Model file for the job. Use its own axes, mm. A direction names the side the tool comes from. Give positions to 0.01 mm unless a question says otherwise; leave off trailing zeros. Order: outer loops, then holes, each group sorted by start corner. A loop starts at its lowest first (then second) coordinate and runs counter-clockwise, first axis right, second up. Notation, with made-up numbers: M 87.25,36 L 114.25,36 A22 cw 114.25,59 Z; hole C 53.25,86 d3. An arc over 180 degrees is marked long. Return JSON: item names as keys, results as strings. Group by question number.
1. Wall check: probe 1 along Z at (x, y) = (55.5, 64); probe 2 along Y at (x, z) = (148.5, 54.5); probe 3 along Y at (x, z) = (10, 7.5). Give the ranges that are in metal, low to high. Write a range as [from, to].
2. Slice it at B-B on x = 24. List the corners of the cut face in (y, z), then the cut area to 3 significant figures.
3. Slice it at A-A on z = 68. List the corners of the cut face in (x, y), then the cut area to 3 significant figures.
4. Two-plate mould, pull along Y, no slides. Class faces 3 (the face through (92, 2, 8)), 4 (the face through (92, 0, 50)), 5 (the face through (92, 75, 98)): released by +Y, released by -Y, zero draft, split by the parting line, or undercut.
5. 3-axis set-ups, long thin cutter, end or side, ignore diameter. For faces 1 (the face through (92, 69, 96)), 2 (the face through (0, 73.2, 96.4)): which of +Z, -Z, +X, -X, +Y, -Y reach the whole face in a straight line?
6. Slice it at D-D on z = 89.5. List the corners of the cut face in (x, y).
7. Slice it at C-C on y = 94. List the corners of the cut face in (x, z).
Autodesk Inventor part; units mm, degrees
ref_plane "YZ Plane" through (0, 0, 0) normal (1, 0, 0) x (0, 1, 0)
ref_plane "XZ Plane" through (0, 0, 0) normal (0, 1, 0) x (-1, 0, 0)
ref_plane "XY Plane" through (0, 0, 0) normal (0, 0, 1) x (1, 0, 0)
sketch "Sketch1" plane through (0, 0, 0) normal (1, 0, 0) x (0, 1, 0)
  line L0 (0, 0) -> (147, 0)
  line L1 (147, 0) -> (147, 98)
  line L2 (147, 98) -> (0, 98)
  line L3 (0, 98) -> (0, 0)
  line L4 (2, 2) -> (145, 2)
  line L5 (145, 2) -> (145, 96)
  line L6 (145, 96) -> (2, 96)
  line L7 (2, 96) -> (2, 2)
  line L8 (137, 96) -> (135, 96)
  line L9 (135, 96) -> (135, 93)
  line L10 (135, 93) -> (137, 93)
  line L11 (137, 93) -> (137, 96)
  circle A0 centre (136, 90.1716) radius 3
  line L12 (135, 2) -> (133, 2)
  line L13 (133, 2) -> (133, 5)
  line L14 (133, 5) -> (135, 5)
  line L15 (135, 5) -> (135, 2)
  circle A1 centre (134, 7.8284) radius 3
  line L16 (2, 84) -> (8, 84)
  line L17 (8, 84) -> (8, 82)
  line L18 (8, 82) -> (2, 82)
  line L19 (2, 82) -> (2, 84)
  line L20 (2, 14) -> (8, 14)
  line L21 (8, 14) -> (8, 16)
  line L22 (8, 16) -> (2, 16)
  line L23 (2, 16) -> (2, 14)
  line L24 (41, 2) -> (43, 2)
  line L25 (43, 2) -> (43, 5)
  line L26 (43, 5) -> (41, 5)
  line L27 (41, 5) -> (41, 2)
  circle A2 centre (10.8284, 83) radius 3
  circle A3 centre (10.8284, 15) radius 3
  circle A4 centre (42, 7.8284) radius 3
  point P0 (2, 16)
  dimension "d36" = 2
  dimension "d37" = 2
  dimension "d38" = 2
  dimension "d39" = 2
  dimension "d40" = 98
  dimension "d41" = 147
  dimension "d42" = 2
  dimension "d43" = 3
  dimension "d44" = 6
  dimension "d45" = 11
  dimension "d46" = 3
  dimension "d47" = 2
  dimension "d48" = 6
  dimension "d49" = 11
  dimension "d50" = 2
  dimension "d51" = 2
  dimension "d52" = 6
  dimension "d53" = 2
  dimension "d54" = 3
  dimension "d55" = 6
  dimension "d56" = 6
  dimension "d57" = 6
  dimension "d58" = 15
  dimension "d60" = 15
  dimension "d61" = 42
extrude "Extrusion1" add sketch "Sketch1" along normal blind 187 contours L3 L2 L1 L0 | L27 A4 L25 L4 | L7 L22 A3 L20 | A4 L26 | L26 A4 | A3 L21 | L21 A3 | L13 A1 L15 L4 | L7 L16 A2 L18 | A1 L14 | L14 A1 | A2 L17 | L17 A2 | L6 L11 A0 L9 | A0 L10 | L10 A0
equation "\"d37\" = d36"
equation "\"d38\" = d36"
equation "\"d39\" = d36"
equation "\"d46\" = d43"
equation "\"d47\" = d42"
equation "\"d48\" = d44"
equation "\"d49\" = d45"
equation "\"d50\" = d42"
equation "\"d51\" = d42"
equation "\"d53\" = d42"
equation "\"d54\" = d43"
equation "\"d55\" = d44"
equation "\"d56\" = d44"
equation "\"d57\" = d44"
properties part number "shell"
Result:
{
 "1": {"probe 1": "z = [0, 2], [96, 98]", "probe 2": "y = [0, 2], [145, 147]", "probe 3": "y = [0, 2], [39.02, 44.98], [131.02, 136.98], [145, 147]"},
 "2": {"outline": "M 0,0 L 147,0 L 147,98 L 0,98 Z; hole M 2,2 L 41,2 L 41,5 A3 cw long 43,5 L 43,2 L 133,2 L 133,5 A3 cw long 135,5 L 135,2 L 145,2 L 145,96 L 137,96 L 137,93 A3 cw long 135,93 L 135,96 L 2,96 L 2,84 L 8,84 A3 cw long 8,82 L 2,82 L 2,16 L 8,16 A3 cw long 8,14 L 2,14 Z", "area": "1,150 mm2"},
 "3": {"outline": "M 0,0 L 187,0 L 187,2 L 0,2 Z; M 0,145 L 187,145 L 187,147 L 0,147 Z", "area": "748 mm2"},
 "4": {"face 3": "undercut", "face 4": "released by -Y", "face 5": "zero draft"},
 "5": {"face 1": "+X, -X", "face 2": "+Z, -Z, -X, +Y, -Y"},
 "6": {"outline": "M 0,0 L 187,0 L 187,2 L 0,2 Z; M 0,133.08 L 187,133.08 L 187,138.92 L 0,138.92 Z; M 0,145 L 187,145 L 187,147 L 0,147 Z"},
 "7": {"outline": "M 0,0 L 187,0 L 187,2 L 0,2 Z; M 0,96 L 187,96 L 187,98 L 0,98 Z"}
}
